```python
from build123d import *

# Parameters (mm, degrees)
F0_W     = 76.2
F0_H     = 76.2
F1_DEPTH = 76.2
F2_R     = 19.05
F3_DEPTH = 25.4
F4_R     = 19.05
F5_DEPTH = 25.4
F6_W     = 38.1
F6_H     = 38.1
F7_DEPTH = 38.1


with BuildPart() as f1:
    # F0 (on Front) → F1 (new body)
    with BuildSketch(Plane.XZ):
        with Locations((4.383184, 4.518054)):
            Rectangle(F0_W, F0_H)
    extrude(amount=F1_DEPTH)

    # F2 (on face) → F3 (join)
    with BuildSketch(Plane.XZ.offset(76.2)):
        with Locations((4.383184, 4.518054)):
            Circle(F2_R)
    extrude(amount=F3_DEPTH)

    # F4 (on face) → F5 (cut)
    with BuildSketch(Plane.XY.offset(42.618054)):
        with Locations((4.383184, -38.1)):
            Circle(F4_R)
    extrude(amount=-F5_DEPTH, mode=Mode.SUBTRACT)

    # F6 (on face) → F7 (cut)
    with BuildSketch(Plane(origin=(-33.716816, 0, 0), x_dir=(0, -1, 0), z_dir=(-1, 0, 0))):
        with Locations((38.1, 4.518054)):
            Rectangle(F6_W, F6_H)
    extrude(amount=-F7_DEPTH, mode=Mode.SUBTRACT)


solid = f1.part
```
Geometry check sheet. Reference: the model listing, model coordinates, mm. A direction names the side the tool comes from. Round coordinates to 2 decimals unless told otherwise and drop trailing zeros. Loops run counter-clockwise (first coordinate to the right, second up) from the corner with the lowest first, then second, coordinate; pieces in that order, holes last. Notation, with made-up numbers: (82, 2) -> (124, 2) arc R14 ccw to (124, 15) -> close; hole circle Ø3 at (0, 26.25). An arc over 180 degrees is marked (long way). Use a Markdown table: item, result.
(1) Sectioned sample at A-A (y = -30.5). Enter the section's corners in (x, z).
Calculated:
| item | result |
|---|---|
| outline | (-33.72, -33.58) -> (42.48, -33.58) -> (42.48, 42.62) -> (21.85, 42.62) -> (21.85, 17.22) -> (4.38, 17.22) -> (4.38, -14.53) -> (-33.72, -14.53) -> close; (-33.72, 23.57) -> (-13.09, 23.57) -> (-13.09, 42.62) -> (-33.72, 42.62) -> close |
(2) Go/stop test with flat-tipped pins: P1, Ø4, axis at y = -91.5, z = 9.5, coming from the +X side; P2, Ø16, axis at y = -31.5, z = 2.5, coming from the -X side; P3, Ø4, axis at y = -40, z = 19.5, coming from the -X side. Record where each tip stops, or that it passes through.
Calculated:
| item | result |
|---|---|
| P1 | x = 23.2 |
| P2 | x = 4.38 |
| P3 | x = 23.03 |
(3) Set-up check for faces 5 (the flat face through (12, -38, 17.218)), 6 (the flat face through (-15, -19.05, 4)), 7 (the flat face through (-5, -76.2, 22)): record each of +Z, -Z, +X, -X, +Y, -Y from which the full face is reachable in a straight line by a thin tool's end or side.
Calculated:
| item | result |
|---|---|
| face 5 | +Z, -X |
| face 6 | -X |
| face 7 | -Y |
(4) Scan lines: probe 1 along X at (y, z) = (-38, 25); probe 2 along Z at (x, y) = (-19, -30); probe 3 along Y at (x, z) = (23.5, 39.5). Record each from-to range of solid material in increasing order.
Calculated:
| item | result |
|---|---|
| probe 1 | -33.72 to -14.67, 23.43 to 42.48 |
| probe 2 | -33.58 to -14.53, 23.57 to 42.62 |
| probe 3 | -76.2 to 0 |
(5) Sectioned sample at B-B (z = 10). Enter the section's corners in (x, y).
Calculated:
| item | result |
|---|---|
| outline | (-33.72, -76.2) -> (-13.86, -76.2) -> (-13.86, -101.6) -> (22.63, -101.6) -> (22.63, -76.2) -> (42.48, -76.2) -> (42.48, 0) -> (-33.72, 0) -> (-33.72, -19.05) -> (4.38, -19.05) -> (4.38, -57.15) -> (-33.72, -57.15) -> close |
(6) Sectioned sample at D-D (z = 19). Enter the section's corners in (x, y), then the cut area to 3 significant figures.
Calculated:
| item | result |
|---|---|
| outline | (-33.72, -76.2) -> (-7.99, -76.2) -> (-7.99, -101.6) -> (16.76, -101.6) -> (16.76, -76.2) -> (42.48, -76.2) -> (42.48, 0) -> (-33.72, 0) -> (-33.72, -19.05) -> (4.38, -19.05) arc R19.05 cw to (4.38, -57.15) -> (-33.72, -57.15) -> close |
| area | 4,410 mm² |
(7) Mould release check, pull along X, two halves, no side actions. Record for faces 1 (the flat face through (-33.717, -38, -21)), 2 (the cylindrical face through (22.553, -32.378, 30.096)), 3 (the cylindrical face through (22.553, -88.722, 10.24)), 4 (the flat face through (-23, -38, 23.568)): released by +X, released by -X, zero draft, split by the parting line, or undercut.
Calculated:
| item | result |
|---|---|
| face 1 | released by -X |
| face 2 | undercut |
| face 3 | split by the parting line |
| face 4 | zero draft |
(8) Sectioned sample at C-C (x = -4). Enter the section's corners in (y, z).
Calculated:
| item | result |
|---|---|
| outline | (-101.6, -12.59) -> (-76.2, -12.59) -> (-76.2, -33.58) -> (0, -33.58) -> (0, 42.62) -> (-20.99, 42.62) -> (-20.99, 23.57) -> (-19.05, 23.57) -> (-19.05, -14.53) -> (-57.15, -14.53) -> (-57.15, 23.57) -> (-55.21, 23.57) -> (-55.21, 42.62) -> (-76.2, 42.62) -> (-76.2, 21.62) -> (-101.6, 21.62) -> close |
